from build123d import *

# Parameters (mm, degrees)
F0_W     = 94.0087363124
F0_H     = 91.4413630962
F1_DEPTH = 88.9
F3_D     = 6.7564
F3_DEPTH = 12.7
F3_TIP   = 2.0298273432
F6_R     = 5.08


# Not quite as in the source:
# - the program builds the solid bodies; features that only make, move or delete a surface that nothing else refers to are left out


with BuildPart() as f1:
    # F0 (on Top) → F1 (new body)
    with BuildSketch(Plane.XY):
        Rectangle(F0_W, F0_H)
    extrude(amount=F1_DEPTH)

    # F3
    with Locations(Plane.XY.offset(88.9)):
        with Locations((-34.3043681562, 33.0206815481), (34.3043681562, 33.0206815481), (34.3043681562, -33.0206815481), (-34.3043681562, -33.0206815481)):
            Hole(F3_D / 2, depth=F3_DEPTH)
            with Locations((0, 0, -(F3_DEPTH + F3_TIP / 2))):  # 118° drill point
                Cone(0, F3_D / 2, F3_TIP, mode=Mode.SUBTRACT)

    # F6
    f6_edges = [f1.edges().sort_by_distance(p)[0] for p in [
        (-47.004368, 45.720682, 44.45),
        (-47.004368, -45.720682, 44.45),
        (-47.004368, 0, 0),
        (-47.004368, 0, 88.9),
    ]]
    fillet(f6_edges, radius=F6_R)


solid = f1.part
Check sheet for the modelled part. Datum: model origin and axes. Units: mm. A direction names the side the tool comes from. Coordinates: 2 decimals unless noted, no trailing zeros. Write item = value, one per line. Start each with the question number.
1. Depth check by flat-ended pin: P1, Ø9, axis at x = -34.3, y = -33.02, coming from the -Z side; P2, Ø4, axis at x = 34.3, y = -33.02, coming from the +Z side; P3, Ø5.5, axis at x = -34.3, y = 33.02, coming from the +Z side. Enter the tip coordinate at first touch or a pass-through.
2. Tool access check on faces 1 (the cylindrical face through (-37.527, 34.035, 82.461)), 2 (the cylindrical face through (-45.56, 0.64, 1.53)). Record the directions out of +Z, -Z, +X, -X, +Y, -Y that give a thin tool (end or side, any length) a straight path to the whole face; none if there is none.
3. Draft check along X on faces 3 (the cylindrical face through (-45.56, -44.19, 45.07)), 4 (the conical face through (34.62, 33.515, 74.523)), 5 (the cylindrical face through (-37.527, -32.006, 82.461)), 6 (the flat face through (2, 1, 88.9)). Enter one of: released by +X, released by -X, zero draft, split by the parting line, or undercut.
4. Material ranges on line 1 (Y direction, x = -43, z = 25), recorded low to high.
Responses:
q1.P1 = 0
q1.P2 = 75.37
q1.P3 = 75.83
q2.face_1 = +Z
q2.face_2 = -Z, -X, +Y, -Y
q3.face_3 = released by -X
q3.face_4 = undercut
q3.face_5 = undercut
q3.face_6 = zero draft
q4.line_1 = -45.61 to 45.61
